```python
from build123d import *

# Parameters (mm, degrees)
BOSS_EXTRUDE1_DEPTH = 9.5
SKETCH4_R           = 5
CUT_EXTRUDE1_DEPTH  = 9.5
BOSS_EXTRUDE2_DEPTH = 36.5
SKETCH8_R           = 12
CUT_EXTRUDE2_DEPTH  = 52.719459587


with BuildPart() as part:
    # Sketch3 → Boss-Extrude1 (new body)
    with BuildSketch(Plane.XY):
        with BuildLine():
            Line((-38.935042057, 18.25), (38.935042057, 18.25))
            ThreePointArc((38.935042057, 18.25), (43, 0), (38.935042057, -18.25))
            Line((38.935042057, -18.25), (-38.935042057, -18.25))
            ThreePointArc((-38.935042057, -18.25), (-43, 0), (-38.935042057, 18.25))
        make_face()
    extrude(amount=BOSS_EXTRUDE1_DEPTH)

    # Sketch4 → Cut-Extrude1 (cut)
    with BuildSketch(Plane.XY.offset(9.5)):
        with Locations((-30.95, 0)):
            Circle(SKETCH4_R)
        with Locations((30.95, 0)):
            Circle(SKETCH4_R)
    extrude(amount=-CUT_EXTRUDE1_DEPTH, mode=Mode.SUBTRACT)

    # Sketch7 → Boss-Extrude2 (add)
    with BuildSketch(Plane.XZ.offset(18.25)):
        with BuildLine():
            Line((0, 0), (0, -0.1))
            ThreePointArc((0, -0.1), (-10.940749517, -3.566165959), (-17.889661819, -12.7))
            Line((-17.889661819, -12.7), (-21.089661819, -12.7))
            Line((-21.089661819, -12.7), (-21.089661819, 0))
            Line((-21.089661819, 0), (0, 0))
        make_face()
        with BuildLine():
            Line((0, 18.9), (0, 9.5))
            Line((0, 9.5), (-25.020791354, 9.5))
            ThreePointArc((-25.020791354, 9.5), (-13.364131098, 16.472461259), (0, 18.9))
        make_face()
    boss_extrude2 = extrude(amount=-BOSS_EXTRUDE2_DEPTH)

    # Mirror1: Boss-Extrude2 across plane
    add(boss_extrude2.mirror(Plane(origin=(0, 0, 0), x_dir=(0, 0, 1), z_dir=(1, 0, 0))))

    # Sketch8 → Cut-Extrude2 (cut, through all)
    with BuildSketch(Plane.XY.offset(9.5)):
        with Locations((-30.95, 0)):
            Circle(SKETCH8_R)
    cut_extrude2 = extrude(amount=CUT_EXTRUDE2_DEPTH, mode=Mode.SUBTRACT)

    # Mirror2: Cut-Extrude2 across plane
    add(cut_extrude2.mirror(Plane(origin=(0, 0, 0), x_dir=(0, 0, 1), z_dir=(1, 0, 0))), mode=Mode.SUBTRACT)

    # Sketch9 → Cut-Revolve1 (revolve, cut)
    with BuildSketch(Plane(origin=(0, 0, 0), x_dir=(0, 0, -1), z_dir=(1, 0, 0)), mode=Mode.PRIVATE) as cut_revolve1_sk:
        Polygon((-18.9, 0), (-18.9, 3), (0, 3), (0, 2), (13.728327228, 2), (13.728327228, 0), align=None)
    revolve(cut_revolve1_sk.sketch.rotate(Axis((0, 0, -13.728327228), (0, 0, 1)), 90), axis=Axis((0, 0, -13.728327228), (0, 0, 1)), mode=Mode.SUBTRACT)


solid = part.part
```
CAD build for the part. Positions are in the model's coordinates, mm. A direction names the side the tool comes from. Coordinates: 2 decimals unless noted, no trailing zeros. Order: outer loops, then holes, each group sorted by start corner. A loop starts at its lowest first (then second) coordinate and runs counter-clockwise, first axis right, second up.
(1) Saw through at D-D, the plane x = -33.5. Write the cut outline in (y, z).
Solution:
outline: (-18.25, 0) - (-4.3, 0) - (-4.3, 9.5) - (-18.25, 9.5) - close; (4.3, 0) - (18.25, 0) - (18.25, 9.5) - (4.3, 9.5) - close
(2) Mould opens along X. For faces 1 (the face through (-43, 0, 5)), 2 (the face through (-1, -18.25, 7)), 3 (the face through (-26.18, 1.5, 4.82)) say: released by +X, released by -X, zero draft, split by the parting line, or undercut.
Solution:
face 1: released by -X
face 2: zero draft
face 3: undercut
(3) Drill centre lines: L1, parallel to Y at x = 0, z = 13.75; L2, parallel to Y at x = -30.95, z = 5; L3, parallel to Z at x = 31.5, y = -16. Where is each one in solid material? Low to high.
Solution:
L1: y = -18.25 to -3, 3 to 18.25
L2: y = -18.25 to -5, 5 to 18.25
L3: z = 0 to 9.5
(4) Saw through at A-A, the plane x = 30.95. Write the cut outline in (y, z), and give its area (3 significant figures).
Solution:
outline: (-18.25, 0) - (-5, 0) - (-5, 9.5) - (-18.25, 9.5) - close; (5, 0) - (18.25, 0) - (18.25, 9.5) - (5, 9.5) - close
area: 252 mm2
(5) Pin check, flat tips, straight feed: pin 1 Ø2 at (y, z) = (-7, -5) entering from -X; pin 2 Ø4 at (x, y) = (-16.5, 0) entering from +Z; pin 3 Ø8 at (x, y) = (-30.95, 0) entering from +Z; pin 4 Ø10 at (y, z) = (-4, 15) entering from -X. Stop position of each tip, or through.
Solution:
pin 1: stops at x = -21.09
pin 2: stops at z = 16.02
pin 3: passes through
pin 4: stops at x = -21.95
(6) Which spindle directions (+Z, -Z, +X, -X, +Y, -Y) get a long thin tool onto all of the face, cutting with end or side? Do faces 4 (the face through (33.8, 4.3, 9.5)), 5 (the face through (-34.3, 4.3, 0)), 6 (the face through (21.09, 0, -6)). Say none if no direction does.
Solution:
face 4: +Z, +X
face 5: -Z, -X, +Y, -Y
face 6: -Z, +X, +Y, -Y
(7) Saw through at C-C, the plane z = 11.5. Write the cut outline in (x, y).
Solution:
outline: (-22.53, -18.25) - (22.53, -18.25) - (22.53, -8.55) arc R12 cw to (22.53, 8.55) - (22.53, 18.25) - (-22.53, 18.25) - (-22.53, 8.55) arc R12 cw to (-22.53, -8.55) - close; hole circle Ø6 at (0, 0)
(8) Saw through at B-B, the plane y = 0. Count the separate pieces of the cut face and the enclosed holes in it, and give its area (3 significant figures).
Solution:
separate pieces: 4
enclosed holes: 0
area: 1,010 mm2
